Could you check a few things on this drawing? It's one solid part, dimensions in mm from its lowest x, y, z. Round coordinates to 2 decimals unless told otherwise and drop trailing zeros. Write each loop counter-clockwise with the first axis right and the second up, starting at its lowest first coordinate (ties: lowest second). Pieces come first, ordered by that corner, then holes. Notation, with made-up numbers: (45.25, -34.75) -> (55.25, -34.75) arc R25 ccw to (55.25, -1.75) -> close; hole circle Ø11 at (41, 35). An arc over 180 degrees is marked (long way). Answer in a Markdown table with one row per item. Add a question column.
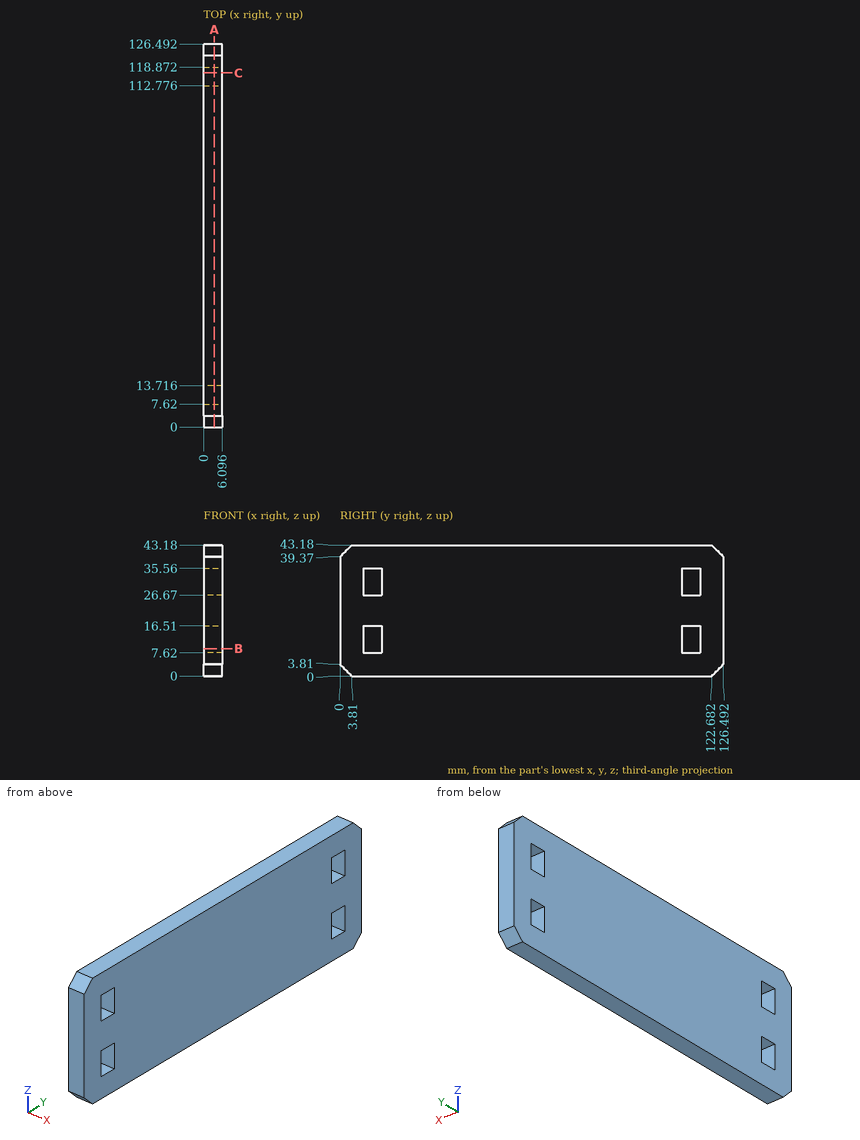
Item 1: If we section it at A-A on x = 3.5: Please give me the cut outline in (y, z), then the cut area to 3 significant figures.
Item 2: I need wall thicknesses on line 1 along Y through (x, z) = (2, 30.5); line 2 along Y through (x, z) = (0.5, 3). Which ranges of each line are inside material? Lowest first, please. Write a range as from..to.
Item 3: If we section it at C-C on y = 117: Please give me the cut outline in (x, z).
Item 4: For P1, Ø2, axis at x = 4.5, y = 79, coming from the -Z side, with a flat end and sliding along its axis, tell me the tip position at first contact or that it passes through.
Item 5: If we section it at B-B on z = 9: Please give me the cut outline in (x, y), then the cut area to 3 significant figures.
Results list:
| question | item | result |
|---|---|---|
| 1 | outline | (0, 3.81) -> (3.81, 0) -> (122.68, 0) -> (126.49, 3.81) -> (126.49, 39.37) -> (122.68, 43.18) -> (3.81, 43.18) -> (0, 39.37) -> close; hole (7.62, 7.62) -> (13.72, 7.62) -> (13.72, 16.51) -> (7.62, 16.51) -> close; hole (7.62, 26.67) -> (13.72, 26.67) -> (13.72, 35.56) -> (7.62, 35.56) -> close; hole (112.78, 7.62) -> (118.87, 7.62) -> (118.87, 16.51) -> (112.78, 16.51) -> close; hole (112.78, 26.67) -> (118.87, 26.67) -> (118.87, 35.56) -> (112.78, 35.56) -> close |
| 1 | area | 5,220 mm² |
| 2 | line 1 | 0..7.62, 13.72..112.78, 118.87..126.49 |
| 2 | line 2 | 0.81..125.68 |
| 3 | outline | (0, 0) -> (6.1, 0) -> (6.1, 7.62) -> (0, 7.62) -> close; (0, 16.51) -> (6.1, 16.51) -> (6.1, 26.67) -> (0, 26.67) -> close; (0, 35.56) -> (6.1, 35.56) -> (6.1, 43.18) -> (0, 43.18) -> close |
| 4 | P1 | z = 0 |
| 5 | outline | (0, 0) -> (6.1, 0) -> (6.1, 7.62) -> (0, 7.62) -> close; (0, 13.72) -> (6.1, 13.72) -> (6.1, 112.78) -> (0, 112.78) -> close; (0, 118.87) -> (6.1, 118.87) -> (6.1, 126.49) -> (0, 126.49) -> close |
| 5 | area | 697 mm² |
